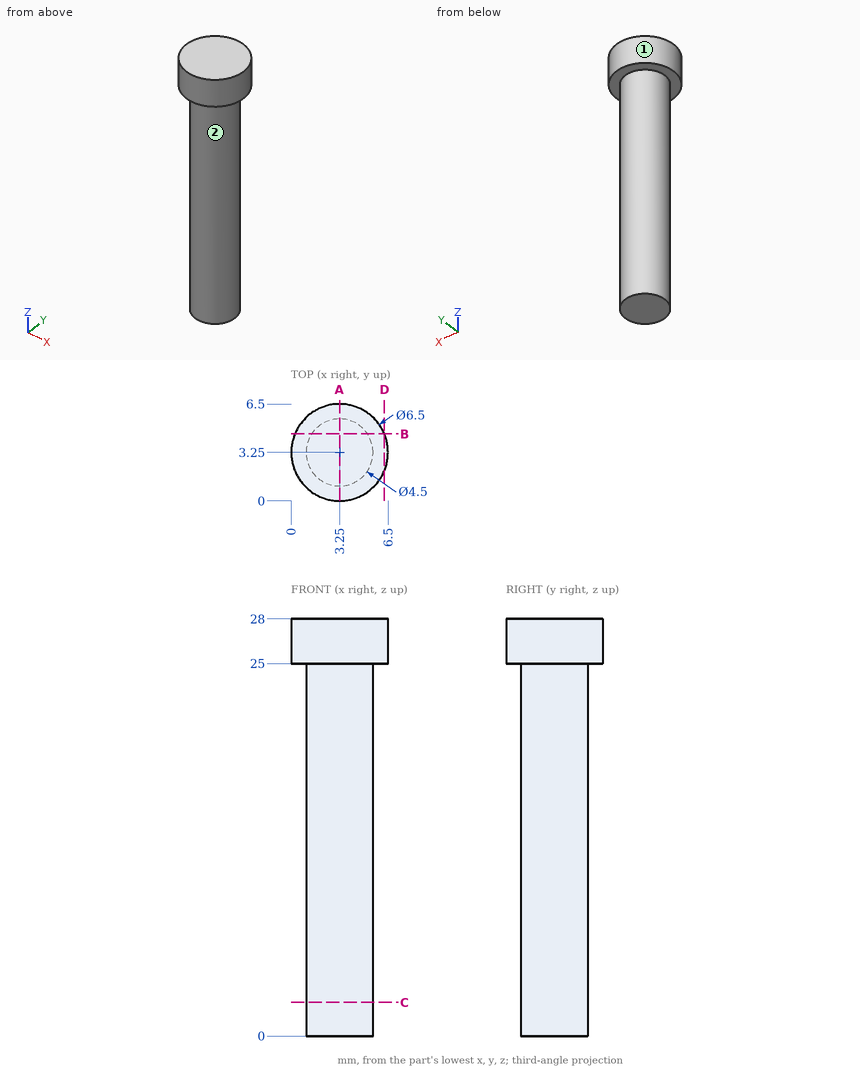
Verification items for this drawing (mm, ordinates from the low corner). A direction names the side the tool comes from. Coordinates: 2 decimals unless noted, no trailing zeros. Order: outer loops, then holes, each group sorted by start corner. A loop starts at its lowest first (then second) coordinate and runs counter-clockwise, first axis right, second up.
Q1. Tool access check on the marked faces 1 and 2. Record the directions out of +Z, -Z, +X, -X, +Y, -Y that give a thin tool (end or side, any length) a straight path to the whole face; none if there is none.
Reply:
face 1: +Z, -Z
face 2: -Z
Q2. Thickness scan on probe 1 along Z at (x, y) = (3.25, 0.5); probe 2 along Y at (x, z) = (3.25, 22.5); probe 3 along Y at (x, z) = (4.25, 10). Record the ranges inside material, lowest first.
Reply:
probe 1: z = 25 to 28
probe 2: y = 1 to 5.5
probe 3: y = 1.23 to 5.27
Q3. Sectioned sample at A-A on x = 3.25. Record the cut outline in (y, z), and give its area (3 significant figures).
Reply:
outline: (0, 25) - (1, 25) - (1, 0) - (5.5, 0) - (5.5, 25) - (6.5, 25) - (6.5, 28) - (0, 28) - close
area: 132 mm2
Q4. Depth check by flat-ended pin: pin 1 Ø1 at (x, y) = (3.5, 2.5) entering from -Z; pin 2 Ø1.5 at (y, z) = (1.5, 6.5) entering from +X; pin 3 Ø1 at (y, z) = (4, 14.5) entering from -X. Enter the tip coordinate at first touch or a pass-through.
Reply:
pin 1: stops at z = 0
pin 2: stops at x = 5.27
pin 3: stops at x = 1.01
Q5. Sectioned sample at C-C on z = 2.25. Record the cut outline in (x, y).
Reply:
outline: circle Ø4.5 at (3.25, 3.25)
Q6. Sectioned sample at B-B on y = 4.5. Record the cut outline in (x, z).
Reply:
outline: (0.25, 25) - (1.38, 25) - (1.38, 0) - (5.12, 0) - (5.12, 25) - (6.25, 25) - (6.25, 28) - (0.25, 28) - close
Q7. Sectioned sample at D-D on x = 6.25. Record the cut outline in (y, z).
Reply:
outline: (2, 25) - (4.5, 25) - (4.5, 28) - (2, 28) - close
